Job drawing, mm, ordinate dimensions from the low corner. One solid piece. Coordinates: 2 decimals unless noted, no trailing zeros. Loops run counter-clockwise (first coordinate to the right, second up) from the corner with the lowest first, then second, coordinate; pieces in that order, holes last. Notation, with made-up numbers: (62, 85.25) - (99, 85.25) arc R14 ccw to (99, 103.25) - close; hole circle Ø7 at (86.5, 15). An arc over 180 degrees is marked (long way). Use a Markdown table: item, result. Add a question column.
1. Band-saw the part on B-B, the plane y = 0.4. Give the cut face in (x, z) (3 decimals).
2. Band-saw the part on D-D, the plane x = 6.5. Give the cut face in (y, z), plus the area to 3 significant figures.
3. Band-saw the part on C-C, the plane z = 6. Give the cut face in (x, y), plus the area to 3 significant figures.
4. Wall check: probe 1 along X at (y, z) = (0.9, 3); probe 2 along X at (y, z) = (0.9, 1.75); probe 3 along X at (y, z) = (0.55, 6.25). Give the ranges that are in metal, low to high. Write a range as [from, to].
5. Band-saw the part on A-A, the plane z = 1.5. Give the cut face in (x, y), plus the area to 3 significant figures.
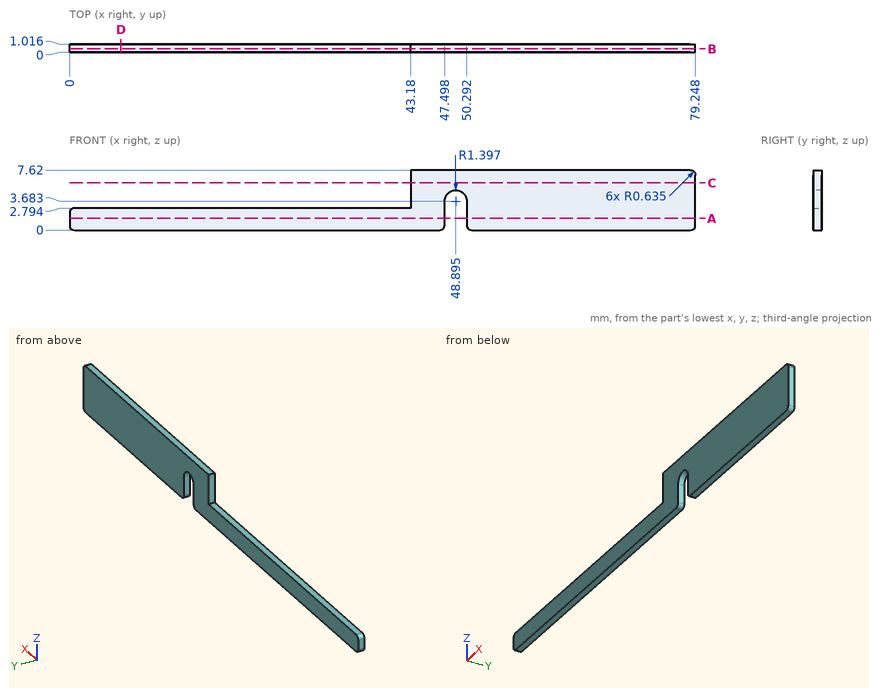
Geometry check:
| question | item | result |
|---|---|---|
| 1 | outline | (0, 0.635) arc R0.635 ccw to (0.635, 0) - (46.863, 0) arc R0.635 ccw to (47.498, 0.635) - (47.498, 3.683) arc R1.397 cw to (50.292, 3.683) - (50.292, 0.635) arc R0.635 ccw to (50.927, 0) - (78.613, 0) arc R0.635 ccw to (79.248, 0.635) - (79.248, 6.985) arc R0.635 ccw to (78.613, 7.62) - (43.18, 7.62) - (43.18, 2.794) - (0.635, 2.794) arc R0.635 ccw to (0, 2.159) - close |
| 2 | outline | (0, 0) - (1.02, 0) - (1.02, 2.79) - (0, 2.79) - close |
| 2 | area | 2.84 mm^2 |
| 3 | outline | (43.18, 0) - (79.25, 0) - (79.25, 1.02) - (43.18, 1.02) - close |
| 3 | area | 36.6 mm^2 |
| 4 | probe 1 | x = [43.18, 47.5], [50.29, 79.25] |
| 4 | probe 2 | x = [0, 47.5], [50.29, 79.25] |
| 4 | probe 3 | x = [43.18, 79.25] |
| 5 | outline | (0, 0) - (47.5, 0) - (47.5, 1.02) - (0, 1.02) - close; (50.29, 0) - (79.25, 0) - (79.25, 1.02) - (50.29, 1.02) - close |
| 5 | area | 77.7 mm^2 |
